For this review, take the finished solid that the model builds, in its own axes (mm). Give positions to 0.01 mm unless a question says otherwise; leave off trailing zeros. Loops run counter-clockwise (first coordinate to the right, second up) from the corner with the lowest first, then second, coordinate; pieces in that order, holes last.
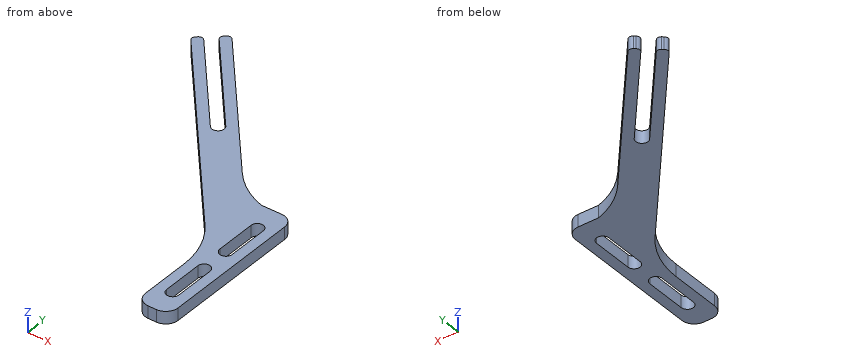
```python
from build123d import *

# Parameters (mm, degrees)
F1_DEPTH    = 3
F2_R        = 1
F3_T1_DEPTH = 3
F4_R        = 3


# Not quite as in the source:
# - a fillet or chamfer that OpenCascade refuses, or shapes differently, is made with other operations: its cross-section is extruded or revolved along the edge and cut away or added


with BuildPart() as f1:
    # F0 (on Top) → F1 (new body)
    with BuildSketch(Plane.XY):
        with BuildLine():
            ThreePointArc((-29.4982599503, 56.7313189632), (-29.6831452005, 54.6180708839), (-31.7963932797, 54.8029561341))
            Line((-31.7963932797, 54.8029561341), (-51.0800215703, 77.7842894277))
            Line((-51.0800215703, 77.7842894277), (-52.9951326781, 76.1773204034))
            Line((-52.9951326781, 76.1773204034), (-8, 22.5542093851))
            Line((-8, 22.5542093851), (-8, 0))
            Line((-8, 0), (0, 0))
            Line((0, 0), (0, 40))
            Line((0, 40), (-8, 40))
            Line((-8, 40), (-8, 35))
            Line((-8, 35), (-46.8667771331, 81.3196212809))
            Line((-46.8667771331, 81.3196212809), (-48.7818882409, 79.7126522567))
            Line((-48.7818882409, 79.7126522567), (-29.4982599503, 56.7313189632))
        make_face()
        with BuildLine():
            Line((-2.5, 16.5), (-2.5, 6.5))
            ThreePointArc((-2.5, 6.5), (-4, 5), (-5.5, 6.5))
            Line((-5.5, 6.5), (-5.5, 16.5))
            ThreePointArc((-5.5, 16.5), (-4, 18), (-2.5, 16.5))
        make_face(mode=Mode.SUBTRACT)
        with BuildLine():
            Line((-2.5, 33.5), (-2.5, 23.5))
            ThreePointArc((-2.5, 23.5), (-4, 22), (-5.5, 23.5))
            Line((-5.5, 23.5), (-5.5, 33.5))
            ThreePointArc((-5.5, 33.5), (-4, 35), (-2.5, 33.5))
        make_face(mode=Mode.SUBTRACT)
    extrude(amount=F1_DEPTH)

    # F2
    f2_edges = [f1.edges().sort_by_distance(p)[0] for p in [
        (-52.995133, 76.17732, 1.5),
        (-51.080022, 77.784289, 1.5),
        (-48.781888, 79.712652, 1.5),
        (-46.866777, 81.319621, 1.5),
    ]]
    fillet(f2_edges, radius=F2_R)

    # F3: fillet of radius 20 on 2 edges, made by hand

    # F3_s2 → F3_t1 (join)
    with BuildSketch(Plane.XY):
        with BuildLine():
            ThreePointArc((-17.4512262706, 46.2635328624), (-13.1787684603, 42.4479872276), (-8, 40))
            Line((-8, 40), (-8, 35))
            Line((-8, 35), (-17.4512262706, 46.2635328624))
        make_face()
        with BuildLine():
            ThreePointArc((-8, 15.2748046998), (-9.2061475843, 22.1152075663), (-12.6791111376, 28.1305568935))
            Line((-12.6791111376, 28.1305568935), (-8, 22.5542093851))
            Line((-8, 22.5542093851), (-8, 15.2748046998))
        make_face()
    extrude(amount=F3_T1_DEPTH)

    # F4
    f4_edges = [f1.edges().sort_by_distance(p)[0] for p in [
        (0, 40, 1.5),
        (-8, 0, 1.5),
        (0, 0, 1.5),
    ]]
    fillet(f4_edges, radius=F4_R)


solid = f1.part
```
Item 1: Clearance check with flat-ended pins moving along their axes: pin 1 Ø0.9 at (x, z) = (-5.5, 1) entering from +Y; pin 2 Ø1.5 at (x, z) = (-16, 2) entering from +Y; pin 3 Ø1 at (x, z) = (-38.5, 2.5) entering from -Y. State where each tip first meets the part, or that it passes through.
Answer:
pin 1: stops at y = 40
pin 2: stops at y = 45.47
pin 3: stops at y = 58.31
Item 2: For L1, parallel to X at y = 11, z = 1; L2, parallel to X at y = 72, z = 0.4; L3, parallel to Y at x = -38, z = 0.85, list the stretches that pass through material, from the lowest coordinate up.
Answer:
L1: x = -8 to -5.5, -2.5 to 0
L2: x = -49.49 to -46.23, -42.31 to -39.05
L3: y = 58.31 to 62.2, 66.86 to 70.75
Item 3: Take a section at D-D on x = -36. Give the boundary of the cut face in (y, z).
Answer:
outline: (55.92, 0) - (59.81, 0) - (59.81, 3) - (55.92, 3) - close; (64.48, 0) - (68.37, 0) - (68.37, 3) - (64.48, 3) - close
Item 4: Take a section at B-B on x = -4. Give the boundary of the cut face in (y, z), and give its area (3 significant figures).
Answer:
outline: (0, 0) - (5, 0) - (5, 3) - (0, 3) - close; (18, 0) - (22, 0) - (22, 3) - (18, 3) - close; (35, 0) - (40, 0) - (40, 3) - (35, 3) - close
area: 42.0 mm2
Item 5: Take a section at A-A on y = 13. Give the boundary of the cut face in (x, z), and give its area (3 significant figures).
Answer:
outline: (-8, 0) - (-5.5, 0) - (-5.5, 3) - (-8, 3) - close; (-2.5, 0) - (0, 0) - (0, 3) - (-2.5, 3) - close
area: 15.0 mm2
Item 6: Take a section at C-C on z = 1.85. Give the boundary of the cut face in (x, y), and give its area (3 significant figures).
Answer:
outline: (-52.35, 75.41) - (-12.68, 28.13) arc R20 cw to (-8, 15.27) - (-8, 3) arc R3 ccw to (-5, 0) - (-3, 0) arc R3 ccw to (0, 3) - (0, 37) arc R3 ccw to (-3, 40) - (-8, 40) arc R20 cw to (-17.45, 46.26) - (-46.22, 80.55) arc R1 ccw to (-47.63, 80.68) - (-48.02, 80.36) arc R1 ccw to (-48.14, 78.95) - (-29.5, 56.73) arc R1.5 cw to (-31.8, 54.8) - (-50.44, 77.02) arc R1 ccw to (-51.85, 77.14) - (-52.23, 76.82) arc R1 ccw to start; hole (-5.5, 6.5) arc R1.5 ccw to (-2.5, 6.5) - (-2.5, 16.5) arc R1.5 ccw to (-5.5, 16.5) - close; hole (-5.5, 23.5) arc R1.5 ccw to (-2.5, 23.5) - (-2.5, 33.5) arc R1.5 ccw to (-5.5, 33.5) - close
area: 691 mm2
